```python
from build123d import *

# Parameters (mm, degrees)
PIN_BODY_W          = 0.636
PIN_BODY_H          = 0.636
BOSS_EXTRUDE1_DEPTH = 2.54


with BuildPart() as part:
    # pin_body → Boss-Extrude1 (new body)
    with BuildSketch(Plane.XY):
        Polygon((0, 2.146446609), (0, 0.353553391), (0.353553391, 0), (0, -0.353553391), (0, -2.146446609), (0.353553391, -2.5), (2.187446609, -2.5), (2.541, -2.146446609), (2.541, -0.353553391), (2.187446609, 0), (2.541, 0.353553391), (2.541, 2.146446609), (2.187446609, 2.5), (2.541, 2.853553391), (2.541, 4.646446609), (2.187446609, 5), (2.541, 5.353553391), (2.541, 7.146446609), (2.187446609, 7.5), (2.541, 7.853553391), (2.541, 9.646446609), (2.187446609, 10), (2.541, 10.353553391), (2.541, 12.146446609), (2.187446609, 12.5), (0.353553391, 12.5), (0, 12.146446609), (0, 10.353553391), (0.353553391, 10), (0, 9.646446609), (0, 7.853553391), (0.353553391, 7.5), (0, 7.146446609), (0, 5.353553391), (0.353553391, 5), (0, 4.646446609), (0, 2.853553391), (0.353553391, 2.5), align=None)
        with Locations((1.2705, -1.25)):
            Rectangle(PIN_BODY_W, PIN_BODY_H, mode=Mode.SUBTRACT)
        with Locations((1.2705, 1.25)):
            Rectangle(PIN_BODY_W, PIN_BODY_H, mode=Mode.SUBTRACT)
        with Locations((1.2705, 3.75)):
            Rectangle(PIN_BODY_W, PIN_BODY_H, mode=Mode.SUBTRACT)
        with Locations((1.2705, 6.25)):
            Rectangle(PIN_BODY_W, PIN_BODY_H, mode=Mode.SUBTRACT)
        with Locations((1.2705, 8.75)):
            Rectangle(PIN_BODY_W, PIN_BODY_H, mode=Mode.SUBTRACT)
        with Locations((1.2705, 11.25)):
            Rectangle(PIN_BODY_W, PIN_BODY_H, mode=Mode.SUBTRACT)
    extrude(amount=BOSS_EXTRUDE1_DEPTH)


solid = part.part
```
The model under review builds one solid part; all positions refer to its coordinate system, in mm. Give positions to 0.01 mm unless a question says otherwise; leave off trailing zeros. Loops run counter-clockwise (first coordinate to the right, second up) from the corner with the lowest first, then second, coordinate; pieces in that order, holes last. Notation, with made-up numbers: (41, 73) - (86, 73) arc R18 ccw to (86, 108) - close; hole circle Ø9 at (62, 78). An arc over 180 degrees is marked (long way). Answer as a JSON object with one key per item and string values.
Q1. Add section A-A on x = 1.15. State the section outline as (y, z) points.
Worked out:
{"outline": "(-2.5, 0) - (-1.57, 0) - (-1.57, 2.54) - (-2.5, 2.54) - close; (-0.93, 0) - (0.93, 0) - (0.93, 2.54) - (-0.93, 2.54) - close; (1.57, 0) - (3.43, 0) - (3.43, 2.54) - (1.57, 2.54) - close; (4.07, 0) - (5.93, 0) - (5.93, 2.54) - (4.07, 2.54) - close; (6.57, 0) - (8.43, 0) - (8.43, 2.54) - (6.57, 2.54) - close; (9.07, 0) - (10.93, 0) - (10.93, 2.54) - (9.07, 2.54) - close; (11.57, 0) - (12.5, 0) - (12.5, 2.54) - (11.57, 2.54) - close"}
Q2. Add section C-C on z = 1.9. Count the separate pieces of the cut face and the enclosed holes in it, plus the area to 3 significant figures.
Worked out:
{"separate pieces": "1", "enclosed holes": "6", "area": "34.2 mm^2"}
Q3. To check wall thickness, follow line 1 along Y through (x, z) = (2.35, 2); line 2 along X through (y, z) = (11.5, 0.25); line 3 along Y through (x, z) = (2.3, 0.35). State the ranges of each line that lie inside material, in increasing order.
Worked out:
{"line 1": "y = -2.34 to -0.16, 0.16 to 2.34, 2.66 to 4.84, 5.16 to 7.34, 7.66 to 9.84, 10.16 to 12.34", "line 2": "x = 0 to 0.95, 1.59 to 2.54", "line 3": "y = -2.39 to -0.11, 0.11 to 2.39, 2.61 to 4.89, 5.11 to 7.39, 7.61 to 9.89, 10.11 to 12.39"}
Q4. Add section B-B on y = 8.75. State the section outline as (x, z) points, plus the area to 3 significant figures.
Worked out:
{"outline": "(0, 0) - (0.95, 0) - (0.95, 2.54) - (0, 2.54) - close; (1.59, 0) - (2.54, 0) - (2.54, 2.54) - (1.59, 2.54) - close", "area": "4.84 mm^2"}
